Study the drawing (mm; zero at the part's minimum x, y, z) and answer. A direction names the side the tool comes from. Give positions to 0.01 mm unless a question says otherwise; leave off trailing zeros. Order: outer loops, then holes, each group sorted by start corner. A loop starts at its lowest first (then second) coordinate and runs counter-clockwise, first axis right, second up. Notation, with made-up numbers: (13, -13.75) - (46, -13.75) arc R19 ccw to (46, 19.25) - close; hole circle Ø9 at (86.5, -20). An arc over 180 degrees is marked (long way). Return JSON: item names as keys, results as strings.
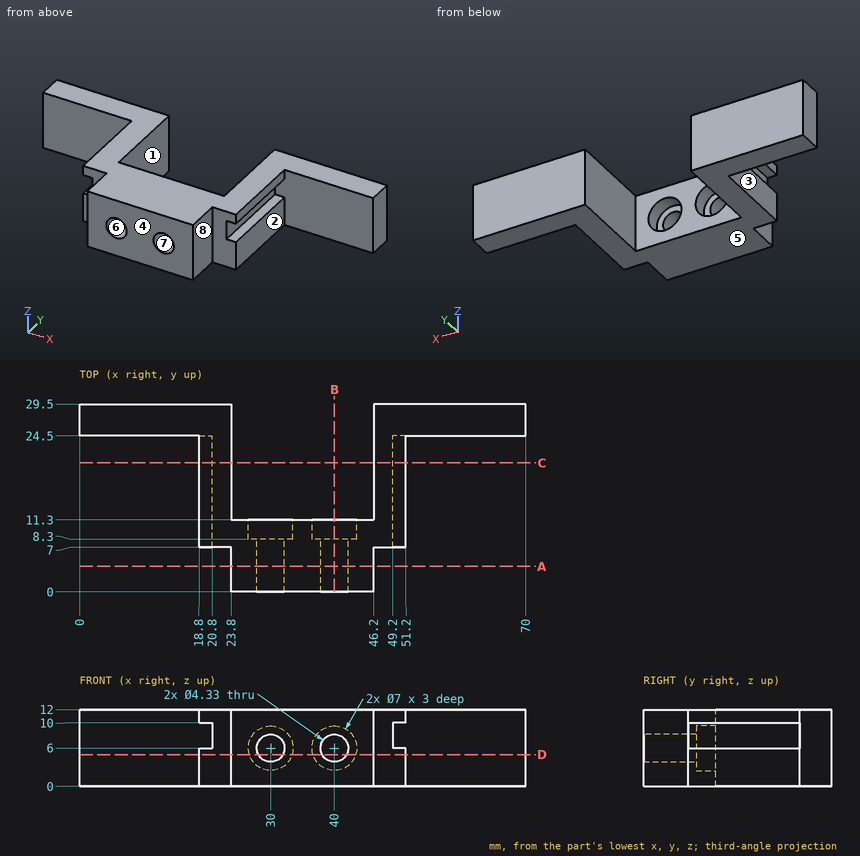
Q1. A cutting plane is placed at A-A (y = 4). Write down the section's boundary in (x, z) (3 decimals), and give its area (3 significant figures).
Values:
{"outline": "(23.8, 0) - (46.2, 0) - (46.2, 12) - (23.8, 12) - close; hole circle Ø4.33 at (30, 6); hole circle Ø4.33 at (40, 6)", "area": "239 mm²"}
Q2. A cutting plane is placed at B-B (x = 40). Write down the section's boundary in (y, z) (3 decimals), and give its area (3 significant figures).
Values:
{"outline": "(0, 0) - (11.3, 0) - (11.3, 2.5) - (8.3, 2.5) - (8.3, 3.835) - (0, 3.835) - close; (0, 8.165) - (8.3, 8.165) - (8.3, 9.5) - (11.3, 9.5) - (11.3, 12) - (0, 12) - close", "area": "78.7 mm²"}
Q3. Consider L1, parallel to X at y = 12.5, z = 7; L2, parallel to X at y = 22.75, z = 4; L3, parallel to X at y = 7.75, z = 6.5. Determine where each line is inside the solid, lowest interval first.
Values:
{"L1": "x = 20.8 to 23.8, 46.2 to 49.2", "L2": "x = 18.8 to 23.8, 46.2 to 51.2", "L3": "x = 20.8 to 27.89, 32.11 to 37.89, 42.11 to 49.2"}
Q4. For the marked faces 1, 2, 3 and 4, determine the directions among +Z, -Z, +X, -X, +Y, -Y from which every point of the face is accessible in a straight line to the end or side of a thin tool.
Values:
{"face 1": "+Z, -Z, +Y", "face 2": "+Z, -Z, +X, -Y", "face 3": "+Z, -Z, -X, -Y", "face 4": "+Z, -Z, +X, -X, -Y"}
Q5. Determine the mould class of the marked faces 5, 6, 7 and 8 for opening direction Z: released by +Z, released by -Z, zero draft, split by the parting line, or undercut.
Values:
{"face 5": "released by -Z", "face 6": "undercut", "face 7": "undercut", "face 8": "zero draft"}
Q6. Given pin 1 (2 mm diameter, centred on x = 25.5, z = 3, fed in from +Y); pin 2 (3 mm diameter, centred on x = 52, y = 4, fed in from -Z); pin 3 (2.5 mm diameter, centred on x = 47.5, z = 8.5, fed in from -Y); pin 4 (1 mm diameter, centred on y = 13.5, z = 10.5, fed in from -X), each flat-ended and moving along its own axis, determine where each tip first touches the part or whether it passes through.
Values:
{"pin 1": "stops at y = 11.3", "pin 2": "passes through", "pin 3": "stops at y = 7", "pin 4": "stops at x = 18.8"}
Q7. A cutting plane is placed at D-D (z = 5). Give the number of separate pieces and of enclosed holes in the cut face, and give its area (3 significant figures).
Values:
{"separate pieces": "3", "enclosed holes": "0", "area": "562 mm²"}
Q8. A cutting plane is placed at C-C (y = 20.25). Write down the section's boundary in (x, z), and give its area (3 significant figures).
Values:
{"outline": "(18.8, 0) - (23.8, 0) - (23.8, 12) - (18.8, 12) - (18.8, 10) - (20.8, 10) - (20.8, 6) - (18.8, 6) - close; (46.2, 0) - (51.2, 0) - (51.2, 6) - (49.2, 6) - (49.2, 10) - (51.2, 10) - (51.2, 12) - (46.2, 12) - close", "area": "104 mm²"}
